```python
from build123d import *

# Parameters (mm, degrees)
F0_W     = 20
F0_H     = 80
F1_DEPTH = 2
F2_DEPTH = 4


with BuildPart() as f1:
    # F0 (on Top) → F1 (new body)
    with BuildSketch(Plane.XY):
        Polygon((-11, -28.898979), (-11, 35.101021), (-15, 15.505103), align=None)
        Rectangle(F0_W, F0_H)
        Polygon((15, 15.505103), (11, 35.101021), (11, -28.898979), align=None)
        Polygon((11, 35.101021), (10, 40), (10, -40), (11, -28.898979), align=None)
        Polygon((-10, -40), (-10, 40), (-11, 35.101021), (-11, -28.898979), align=None)
    extrude(amount=F1_DEPTH)

    # F0 (on Top) → F2 (join)
    with BuildSketch(Plane.XY):
        Polygon((-15, 15.505103), (-11, 35.101021), (-11, 41), (-16.125, 15.89273), (-11, -41), (-11, -28.898979), align=None)
        Polygon((-10, 40), (10, 40), (11, 35.101021), (11, 41), (-11, 41), (-11, 35.101021), align=None)
        Polygon((11, 41), (11, 35.101021), (15, 15.505103), (11, -28.898979), (11, -41), (16.125, 15.89273), align=None)
        Polygon((11, -28.898979), (10, -40), (-10, -40), (-11, -28.898979), (-11, -41), (11, -41), align=None)
    extrude(amount=F2_DEPTH)


solid = f1.part
```
The model under review builds one solid part; all positions refer to its coordinate system, in mm. A direction names the side the tool comes from. Round coordinates to 2 decimals unless told otherwise and drop trailing zeros. Loops run counter-clockwise (first coordinate to the right, second up) from the corner with the lowest first, then second, coordinate; pieces in that order, holes last. Notation, with made-up numbers: (22, -17) - (38, -17) arc R11 ccw to (38, -10) - close; hole circle Ø7 at (47, 86). An arc over 180 degrees is marked (long way). Use a Markdown table: item, result. Add a question column.
Q1. Add section C-C (x = 8). State the section outline as (y, z) points.
Q2. Machinability: for faces 4 (the face through (0, 1, 2)), 5 (the face through (0, -41, 2)), which of the approach directions +Z, -Z, +X, -X, +Y, -Y give a long, thin tool a straight path to every point of the face, cutting with its end or side? Answer none if there is none.
Q3. For probe 1 along Y at (x, z) = (8, 2.2); probe 2 along Z at (x, y) = (10, 22); probe 3 along X at (y, z) = (-31, 2.8), list the stretches that pass through material, from the lowest coordinate up.
Q4. The part is to be moulded in two halves that separate along X. For faces 1 (the face through (-13.598, -12.155, 1.972)), 2 (the face through (0, 40, 3)), 3 (the face through (13.527, -12.952, 1.972)), say which applies: pulls with the +X half, pulls with the -X half, needs draft (parallel to the pull), parting line crosses it, or undercut.
Q5. Insertion check: pin 1 Ø9 at (x, y) = (7, -12.5) entering from +Z. The pin has a flat end and moves straight along its axis. Give the tip position at first contact, or say it passes through.
Q6. Add section A-A (z = 2.65). State the section outline as (x, y) points (3 decimals).
Q7. Add section B-B (y = 5.5). State the section outline as (x, z) points, plus the area to 3 significant figures.
Worked answers:
| question | item | result |
|---|---|---|
| 1 | outline | (-41, 0) - (41, 0) - (41, 4) - (40, 4) - (40, 2) - (-40, 2) - (-40, 4) - (-41, 4) - close |
| 2 | face 4 | +Z |
| 2 | face 5 | +Z, -Z, +X, -X, -Y |
| 3 | probe 1 | -41 to -40, 40 to 41 |
| 3 | probe 2 | 0 to 2 |
| 3 | probe 3 | -11.9 to -10.81, 10.81 to 11.9 |
| 4 | face 1 | pulls with the -X half |
| 4 | face 2 | undercut |
| 4 | face 3 | pulls with the +X half |
| 5 | pin 1 | z = 2 |
| 6 | outline | (-16.125, 15.893) - (-11, -41) - (11, -41) - (16.125, 15.893) - (11, 41) - (-11, 41) - close; hole (-15, 15.505) - (-10, -40) - (10, -40) - (15, 15.505) - (10, 40) - (-10, 40) - close |
| 7 | outline | (-15.19, 0) - (15.19, 0) - (15.19, 4) - (14.1, 4) - (14.1, 2) - (-14.1, 2) - (-14.1, 4) - (-15.19, 4) - close |
| 7 | area | 65.1 mm² |
